from build123d import *

# Parameters (mm, degrees)
F2_DEPTH = 0.25
F4_DEPTH = 0.5
F0_R     = 8.255
F6_DEPTH = 2.5
F7_R     = 0.2


with BuildPart() as f2:
    # F1 (on Top) → F2 (new body, symmetric)
    with BuildSketch(Plane.XY):
        Polygon((-9, -2.4115427319), (-6.5884572681, -6.5884572681), (-2.4115427319, -9), (2.4115427319, -9), (6.5884572681, -6.5884572681), (9, -2.4115427319), (9, 2.4115427319), (6.5884572681, 6.5884572681), (2.4115427319, 9), (-2.4115427319, 9), (-6.5884572681, 6.5884572681), (-9, 2.4115427319), align=None)
    extrude(amount=F2_DEPTH, both=True)

    # F3 (on face) → F4 (join)
    with BuildSketch(Plane.XY.offset(0.25)):
        Polygon((-8.0691792495, 4.6587428118), (-9.3174856237, 0), (-8.0691792495, -4.6587428118), (-4.6587428118, -8.0691792495), (0, -9.3174856237), (4.6587428118, -8.0691792495), (8.0691792495, -4.6587428118), (9.3174856237, 0), (8.0691792495, 4.6587428118), (4.6587428118, 8.0691792495), (0, 9.3174856237), (-4.6587428118, 8.0691792495), align=None)
    extrude(amount=F4_DEPTH)

    # F5: F2 across plane


with BuildPart() as f2_1:
    add(f2.part)
    add(f2.part.mirror(Plane.XY))

    # F0 (on Top) → F6 (cut, symmetric)
    with BuildSketch(Plane.XY):
        Circle(F0_R)
    extrude(amount=F6_DEPTH, both=True, mode=Mode.SUBTRACT)

    # F7
    f7_edges = [f2_1.edges().sort_by_distance(p)[0] for p in [
        (-8.255, 0, -0.75),
        (8.255, 0, 0),
        (-8.255, 0, 0.75),
    ]]
    fillet(f7_edges, radius=F7_R)


solid = f2_1.part
The model under review builds one solid part; all positions refer to its coordinate system, in mm. A direction names the side the tool comes from. Give positions to 0.01 mm unless a question says otherwise; leave off trailing zeros. Write each loop counter-clockwise with the first axis right and the second up, starting at its lowest first coordinate (ties: lowest second). Pieces come first, ordered by that corner, then holes.
1. Wall thickness on L1, parallel to Y at x = 0, z = 0 (3 decimals); L2, parallel to X at y = 1.75, z = 0.15; L3, parallel to Y at x = -5, z = 0.3: over which ranges is each line inside the solid? List them lowest first.
2. Add section A-A, the plane z = 0. Write out the cut boundary in (x, y) (3 decimals).
3. Tool access review of faces 4 (the flat face through (-2.3, 8.7, -0.5)), 5 (the flat face through (8.7, 2.3, 0.5)), 6 (the flat face through (2.362, 8.685, -0.496)): name each direction out of +Z, -Z, +X, -X, +Y, -Y from which nothing blocks a thin tool from reaching the whole face with its end or side.
4. Draft analysis for pull direction Z (two halves, no side actions). For faces 1 (the flat face through (-4.529, -7.777, 0.004)), 2 (the flat face through (8.7, 2.3, -0.5)), 3 (the flat face through (-7.777, 4.529, 0.004)), state which applies: +Z half, -Z half, draft (parallel to the pull), parting line (faces both ways), or undercut.
5. For P1, Ø0.6, axis at x = -5, y = 8, coming from the -Z side, flat-tipped, find the tip position at first contact; note if it passes through.
Worked answers:
1. L1: y = -9 to -8.255, 8.255 to 9
1. L2: x = -9 to -8.07, 8.07 to 9
1. L3: y = -7.73 to -6.57, 6.57 to 7.73
2. outline: (-9, -2.412) - (-6.588, -6.588) - (-2.412, -9) - (2.412, -9) - (6.588, -6.588) - (9, -2.412) - (9, 2.412) - (6.588, 6.588) - (2.412, 9) - (-2.412, 9) - (-6.588, 6.588) - (-9, 2.412) - close; hole circle Ø16.51 at (0, 0)
3. face 4: -Z, -X, +Y
3. face 5: +Z, +X, +Y
3. face 6: -Z, +X, +Y
4. face 1: undercut
4. face 2: draft
4. face 3: undercut
5. P1: stops at z = -0.75
